from build123d import *

# Parameters (mm, degrees)
SKETCH1_W           = 40
SKETCH1_H           = 40
BOSS_EXTRUDE1_DEPTH = 1
SKETCH1_3_W         = 45
SKETCH1_3_H         = 45
SKETCH1_3_W_2       = 40
SKETCH1_3_H_2       = 40
BOSS_EXTRUDE2_DEPTH = 6
FILLET1_R           = 3


with BuildPart() as part:
    # Sketch1 → Boss-Extrude1 (new body)
    with BuildSketch(Plane(origin=(0, 0, 0), x_dir=(1, 0, 0), z_dir=(0, 1, 0))):
        Rectangle(SKETCH1_W, SKETCH1_H)
    extrude(amount=BOSS_EXTRUDE1_DEPTH)

    # Sketch1<3> → Boss-Extrude2 (add)
    with BuildSketch(Plane(origin=(0, 0, 0), x_dir=(1, 0, 0), z_dir=(0, 1, 0))):
        Rectangle(SKETCH1_3_W, SKETCH1_3_H)
        Rectangle(SKETCH1_3_W_2, SKETCH1_3_H_2, mode=Mode.SUBTRACT)
    extrude(amount=BOSS_EXTRUDE2_DEPTH)

    # Fillet1
    fillet1_edges = [part.edges().sort_by_distance(p)[0] for p in [
        (22.5, 3, 22.5),
        (22.5, 3, -22.5),
        (-22.5, 3, -22.5),
        (-22.5, 3, 22.5),
        (20, 3.5, -20),
        (-20, 3.5, -20),
        (-20, 3.5, 20),
        (20, 3.5, 20),
    ]]
    fillet(fillet1_edges, radius=FILLET1_R)


solid = part.part
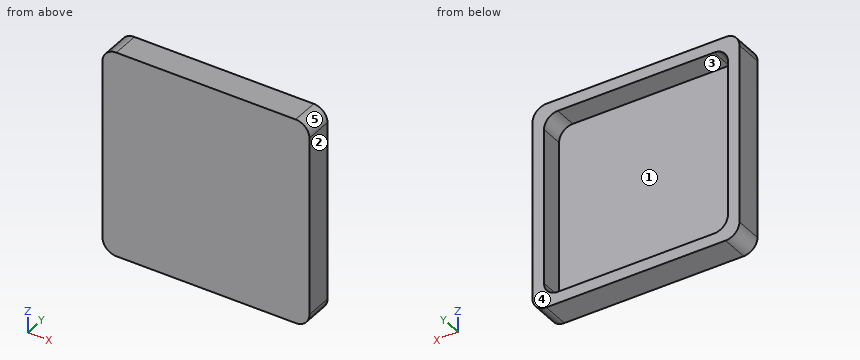
Verification items for the finished model (mm, model axes). Face numbers are marked on the shaded views. A direction names the side the tool comes from. Round coordinates to 2 decimals unless told otherwise and drop trailing zeros. Loops run counter-clockwise (first coordinate to the right, second up) from the corner with the lowest first, then second, coordinate; pieces in that order, holes last. Notation, with made-up numbers: (-11.5, 39.25) - (46.5, 39.25) arc R13 ccw to (46.5, 63.25) - close; hole circle Ø3 at (80.25, 2). An arc over 180 degrees is marked (long way). Use a Markdown table: item, result. Add a question column.
1. Section check B-B, the plane y = 3.8. Record the boundary of the cut face in (x, z).
2. Access from +Z, -Z, +X, -X, +Y, -Y to the whole of each face (thin tool, end or side, straight path). Record for the marked faces 1 and 2.
3. Release check for a two-part mould opening along X. For the marked faces 3, 4 and 5 record: released by +X, released by -X, zero draft, split by the parting line, or undercut.
4. Gauge pin test, flat ends, axial feed: pin 1 (5 mm diameter, centred on x = 9, z = -2.5, fed in from -Y); pin 2 (1.5 mm diameter, centred on x = -5, z = 9, fed in from +Y). Record the tip position at first contact, or that the pin passes through.
5. Section check C-C, the plane z = -11. Record the boundary of the cut face in (x, y), plus the area to 3 significant figures.
6. Thickness scan on probe 1 along X at (y, z) = (4.05, -13); probe 2 along Y at (x, z) = (18, 17). Record the ranges inside material, lowest first. Write a range as [from, to].
7. Section check A-A, the plane x = 7. Record the boundary of the cut face in (y, z).
Checks:
| question | item | result |
|---|---|---|
| 1 | outline | (-22.5, -19.5) arc R3 ccw to (-19.5, -22.5) - (19.5, -22.5) arc R3 ccw to (22.5, -19.5) - (22.5, 19.5) arc R3 ccw to (19.5, 22.5) - (-19.5, 22.5) arc R3 ccw to (-22.5, 19.5) - close; hole (-20, -17) arc R3 ccw to (-17, -20) - (17, -20) arc R3 ccw to (20, -17) - (20, 17) arc R3 ccw to (17, 20) - (-17, 20) arc R3 ccw to (-20, 17) - close |
| 2 | face 1 | +Y |
| 2 | face 2 | +Z, -Z, +X, +Y, -Y |
| 3 | face 3 | undercut |
| 3 | face 4 | zero draft |
| 3 | face 5 | released by +X |
| 4 | pin 1 | stops at y = 0 |
| 4 | pin 2 | stops at y = 1 |
| 5 | outline | (-22.5, 0) - (22.5, 0) - (22.5, 6) - (20, 6) - (20, 1) - (-20, 1) - (-20, 6) - (-22.5, 6) - close |
| 5 | area | 70.0 mm^2 |
| 6 | probe 1 | x = [-22.5, -20], [20, 22.5] |
| 6 | probe 2 | y = [0, 1] |
| 7 | outline | (0, -22.5) - (6, -22.5) - (6, -20) - (1, -20) - (1, 20) - (6, 20) - (6, 22.5) - (0, 22.5) - close |
